from build123d import *

# Parameters (mm, degrees)
SKETCH_1_W          = 42
SKETCH_1_H          = 42
EXTRUDE_1_DEPTH     = 48
SKETCH_2_R          = 21
EXTRUDE_2_DEPTH     = 42
SKETCH_3_R          = 12.5
EXTRUDE_3_DEPTH     = 2
EXTRUDE_4_DEPTH     = 18
SKETCH_5_R          = 2
CUT_EXTRUDE_1_DEPTH = 4


with BuildPart() as part:
    # 草图1 → 凸台-拉伸1 (new body)
    with BuildSketch(Plane.XY):
        Rectangle(SKETCH_1_W, SKETCH_1_H)
    extrude(amount=EXTRUDE_1_DEPTH)

    # 草图2 → 凸台-拉伸2 (add)
    with BuildSketch(Plane.XY.offset(48)):
        Circle(SKETCH_2_R)
    extrude(amount=EXTRUDE_2_DEPTH)

    # 草图3 → 凸台-拉伸3 (add)
    with BuildSketch(Plane.XY.offset(90)):
        Circle(SKETCH_3_R)
    extrude(amount=EXTRUDE_3_DEPTH)

    # 草图4 → 凸台-拉伸4 (add)
    with BuildSketch(Plane.XY.offset(92)):
        with BuildLine():
            Line((-2.645751311, 3), (2.645751311, 3))
            ThreePointArc((2.645751311, 3), (0, -4), (-2.645751311, 3))
        make_face()
    extrude(amount=EXTRUDE_4_DEPTH)

    # 草图5 → 切除-拉伸1 (cut)
    with BuildSketch(Plane.XY.offset(90)):
        with Locations((0, -17.5)):
            Circle(SKETCH_5_R)
        with Locations((-17.5, 0)):
            Circle(SKETCH_5_R)
        with Locations((0, 17.5)):
            Circle(SKETCH_5_R)
        with Locations((17.5, 0)):
            Circle(SKETCH_5_R)
    extrude(amount=-CUT_EXTRUDE_1_DEPTH, mode=Mode.SUBTRACT)


solid = part.part
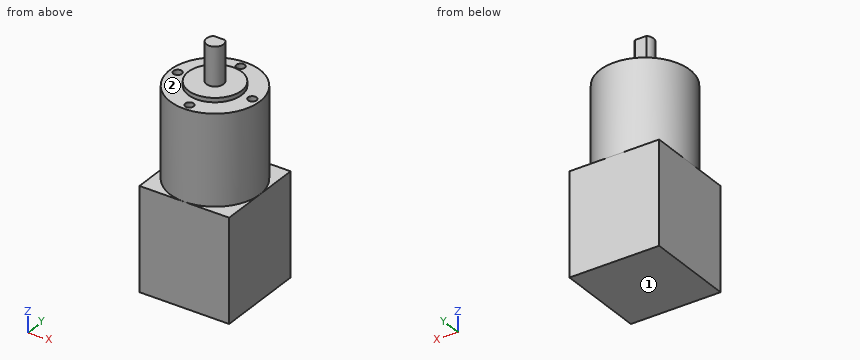
Read the model definition and answer for the solid it produces. Units are mm, in the model's axes. Face numbers are marked on the shaded views. A direction names the side the tool comes from. Coordinates: 2 decimals unless noted, no trailing zeros. Write each loop counter-clockwise with the first axis right and the second up, starting at its lowest first coordinate (ties: lowest second). Pieces come first, ordered by that corner, then holes. Notation, with made-up numbers: M 22.5,-29.75 L 79.5,-29.75 A14 ccw 79.5,-16.75 Z; hole C 54,65.25 d11. An arc over 180 degrees is marked long. Use a Markdown table: item, result.
Q1. Straight lines are drawn through the part: L1, parallel to Y at x = 0, z = 89; L2, parallel to Z at x = 0, y = 10; L3, parallel to Z at x = 4, y = 15.5. For each, find the intervals that lie inside material, in ascending order. Write a range as [from, to].
Answer block:
| item | result |
|---|---|
| L1 | y = [-21, -19.5], [-15.5, 15.5], [19.5, 21] |
| L2 | z = [0, 92] |
| L3 | z = [0, 90] |
Q2. The part is cut by section D-D, the plane z = 102. Write down the section's boundary in (x, y).
Answer block:
| item | result |
|---|---|
| outline | M -2.65,3 A4 ccw long 2.65,3 Z |
Q3. The part is cut by section A-A, the plane x = -7. Write down the section's boundary in (y, z).
Answer block:
| item | result |
|---|---|
| outline | M -21,0 L 21,0 L 21,48 L 19.8,48 L 19.8,90 L 10.36,90 L 10.36,92 L -10.36,92 L -10.36,90 L -19.8,90 L -19.8,48 L -21,48 Z |
Q4. The part is cut by section B-B, the plane z = 73.5. Write down the section's boundary in (x, y), then the cut area to 3 significant figures.
Answer block:
| item | result |
|---|---|
| outline | C 0,0 d42 |
| area | 1,390 mm2 |
Q5. The part is cut by section C-C, the plane y = -17.5. Write down the section's boundary in (x, z).
Answer block:
| item | result |
|---|---|
| outline | M -21,0 L 21,0 L 21,48 L 11.61,48 L 11.61,90 L 2,90 L 2,86 L -2,86 L -2,90 L -11.61,90 L -11.61,48 L -21,48 Z |
Q6. Which of the six approach directions +Z, -Z, +X, -X, +Y, -Y give full straight-line access (tool end or side, diameter ignored) to the marked faces 1 and 2?
Answer block:
| item | result |
|---|---|
| face 1 | -Z, +X, -X, +Y, -Y |
| face 2 | +Z |
Q7. Each of these flat-tipped pins is pushed along its axis until it touches: pin 1 Ø4.5 at (x, y) = (-17.5, -0.5) entering from +Z; pin 2 Ø1.5 at (x, z) = (-14.5, 90.5) entering from +Y; pin 3 Ø2 at (x, y) = (0.5, -18) entering from +Z. Where does it stop, or does it pass through?
Answer block:
| item | result |
|---|---|
| pin 1 | stops at z = 90 |
| pin 2 | stops at y = 15.71 |
| pin 3 | stops at z = 86 |
